The listing builds one solid part. Answer for the finished solid, in the listing's coordinates (mm). Face numbers are marked on the shaded views. A direction names the side the tool comes from. Round coordinates to 2 decimals unless told otherwise and drop trailing zeros. Write each loop counter-clockwise with the first axis right and the second up, starting at its lowest first coordinate (ties: lowest second). Pieces come first, ordered by that corner, then holes.
Item 1: Find the intervals of material crossed by probe 1 along Y at (x, z) = (1.5, -4); probe 2 along Z at (x, y) = (-8.5, 1.6); probe 3 along X at (y, z) = (2.2, 5.25), in increasing order.
Item 2: Each of these flat-tipped pins is pushed along its axis until it touches: pin 1 (4 mm diameter, centred on x = -2.5, z = -7.5, fed in from -Y); pin 2 (5 mm diameter, centred on x = 4.5, z = 7, fed in from +Y); pin 3 (1 mm diameter, centred on x = 3, z = -5, fed in from +Y); pin 4 (8 mm diameter, centred on x = -6, z = 4.5, fed in from +Y). Where does it stop, or does it pass through?
Item 3: A tool of negligible diameter and unlimited length cuts with its end or side. For the marked faces 1, 2, 3, 4 and 5, from which of +Z, -Z, +X, -X, +Y, -Y can it reach the whole face along a straight path? Write none if from no direction.
Item 4: Find section D-D on y = 3.9. Give the vertices of the cut face in (x, z), then the cut area to 3 significant figures.
Item 5: Find section A-A on x = 0.75. Give the vertices of the cut face in (y, z), then the cut area to 3 significant figures.
Item 6: Find section B-B on z = -1.5. Give the vertices of the cut face in (x, y), then the cut area to 3 significant figures.
Item 7: Find section C-C on y = 5.15. Give the vertices of the cut face in (x, z).
```python
from build123d import *

# Parameters (mm, degrees)
SKETCH1_W      = 20
SKETCH1_H      = 20
EXTRUDE1_DEPTH = 1.5
SKETCH2_W      = 20
SKETCH2_H      = 10
EXTRUDE2_DEPTH = 3
SKETCH3_W      = 10
SKETCH3_H      = 10
EXTRUDE3_DEPTH = 1.5
SKETCH4_W      = 10
SKETCH4_H      = 10
EXTRUDE4_DEPTH = 1.5


with BuildPart() as part:
    # Sketch1 → Extrude1 (new body)
    with BuildSketch(Plane(origin=(0, 0, 0), x_dir=(1, 0, 0), z_dir=(0, 1, 0))):
        Rectangle(SKETCH1_W, SKETCH1_H)
    extrude(amount=EXTRUDE1_DEPTH)

    # Sketch2 → Extrude2 (add)
    with BuildSketch(Plane(origin=(0, 1.5, 0), x_dir=(1, 0, 0), z_dir=(0, 1, 0))):
        with Locations((0, 5)):
            Rectangle(SKETCH2_W, SKETCH2_H)
    extrude(amount=EXTRUDE2_DEPTH)

    # Sketch3 → Extrude3 (add)
    with BuildSketch(Plane(origin=(0, 1.5, 0), x_dir=(1, 0, 0), z_dir=(0, 1, 0))):
        with Locations((5, -5)):
            Rectangle(SKETCH3_W, SKETCH3_H)
    extrude(amount=EXTRUDE3_DEPTH)

    # Sketch4 → Extrude4 (add)
    with BuildSketch(Plane(origin=(0, 4.5, 0), x_dir=(-1, 0, 0), z_dir=(0, 1, 0))):
        with Locations((5, -5)):
            Rectangle(SKETCH4_W, SKETCH4_H)
    extrude(amount=EXTRUDE4_DEPTH)


solid = part.part
```
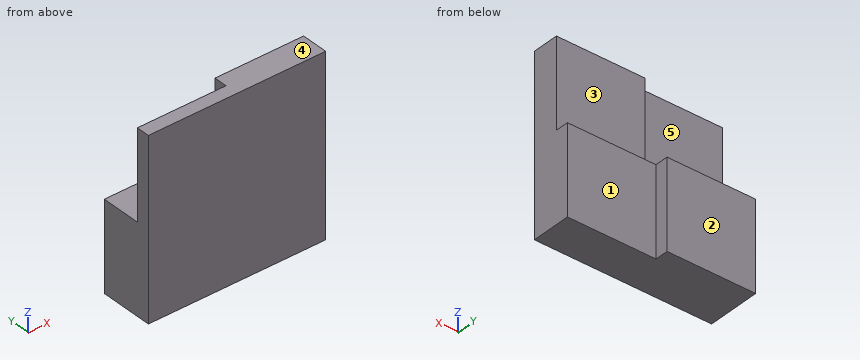
Check values:
1. probe 1: y = 0 to 4.5
1. probe 2: z = -10 to 0
1. probe 3: x = 0 to 10
2. pin 1: stops at y = 0
2. pin 2: stops at y = 3
2. pin 3: stops at y = 4.5
2. pin 4: stops at y = 1.5
3. face 1: +Z, -Z, +X, +Y
3. face 2: +Z, -Z, +X, -X, +Y
3. face 3: +Z, +X, -X, +Y
3. face 4: +Z, +X, -X, +Y, -Y
3. face 5: +Z, -X, +Y
4. outline: (-10, -10) - (10, -10) - (10, 0) - (-10, 0) - close
4. area: 200 mm2
5. outline: (0, -10) - (4.5, -10) - (4.5, 0) - (3, 0) - (3, 10) - (0, 10) - close
5. area: 75.0 mm2
6. outline: (-10, 0) - (10, 0) - (10, 4.5) - (0, 4.5) - (0, 6) - (-10, 6) - close
6. area: 105 mm2
7. outline: (-10, -10) - (0, -10) - (0, 0) - (-10, 0) - close
